Design review of the part built by this model. Coordinates are the model's own, in mm. A direction names the side the tool comes from. Round coordinates to 2 decimals unless told otherwise and drop trailing zeros. Loops run counter-clockwise (first coordinate to the right, second up) from the corner with the lowest first, then second, coordinate; pieces in that order, holes last. Notation, with made-up numbers: (34.25, 84) - (74.25, 84) arc R17 cw to (74.25, 113) - close; hole circle Ø4 at (17.5, -40). An arc over 180 degrees is marked (long way). Return JSON: item names as keys, results as strings. Group by question number.
from build123d import *

# Parameters (mm, degrees)
MAIN_BODY_SKETCH_W            = 29
MAIN_BODY_SKETCH_H            = 11
MAIN_BODY_EXTRUDE_DEPTH       = 1.5
TILTED_OFFSHOOT_SKETCH_W      = 11
TILTED_OFFSHOOT_SKETCH_H      = 24
TILTED_OFFSHOOT_EXTRUDE_DEPTH = 1.5
F_2_7_2_7_DIAMETER_HOLE1_D    = 2.7
F_3_0_3_DIAMETER_HOLE1_D      = 3


with BuildPart() as part:
    # Main Body Sketch → Main Body Extrude (new body)
    with BuildSketch(Plane(origin=(0, 0, 0), x_dir=(1, 0, 0), z_dir=(0, 1, 0))):
        Polygon((-29, -11), (-29, 0), (-29, 2.5), (-47.33030278, 2.5), (-47.33030278, -13.5), (-29, -13.5), align=None)
        with Locations((-14.5, -5.5)):
            Rectangle(MAIN_BODY_SKETCH_W, MAIN_BODY_SKETCH_H)
        with BuildLine():
            ThreePointArc((-47.33030278, -13.5), (-49, -5.5), (-47.33030278, 2.5))
            Line((-47.33030278, 2.5), (-47.33030278, -13.5))
        make_face()
    extrude(amount=MAIN_BODY_EXTRUDE_DEPTH)

    # Tilted Offshoot Sketch → Tilted Offshoot Extrude (add)
    with BuildSketch(Plane(origin=(0, 0, 0), x_dir=(0, 0, 1), z_dir=(-0.707106781, 0.707106781, 0))):
        with Locations((5.5, 12)):
            Rectangle(TILTED_OFFSHOOT_SKETCH_W, TILTED_OFFSHOOT_SKETCH_H)
    extrude(amount=TILTED_OFFSHOOT_EXTRUDE_DEPTH)

    # Ø2.7 (2.7) Diameter Hole1 (through all)
    with Locations(Plane(origin=(0, 1.5, 0), x_dir=(1, 0, 0), z_dir=(0, 1, 0))):
        with Locations((-45, -10.5), (-33, -0.5)):
            Hole(F_2_7_2_7_DIAMETER_HOLE1_D / 2)

    # Ø3.0 (3) Diameter Hole1 (through all)
    with Locations(Plane(origin=(-1.060660172, 1.060660172, 0), x_dir=(0.707106781, 0.707106781, 0), z_dir=(-0.707106781, 0.707106781, 0))):
        with Locations((20, -5.5)):
            Hole(F_3_0_3_DIAMETER_HOLE1_D / 2)


solid = part.part
Q1. Draft analysis for pull direction X (two halves, no side actions). For faces 1 (the flat face through (-29, 1, 12)), 2 (the flat face through (-4, 1, 0)), 3 (the cylindrical face through (-44.005, 0.74, 9.588)), state which applies: pulls with the +X half, pulls with the -X half, needs draft (parallel to the pull), parting line crosses it, or undercut.
Q2. Add section B-B, the plane y = 4.5. State the section outline as (x, z) points.
Q3. For line 1 (Z direction, x = -45, y = 0.4); line 2 (Z direction, x = -33, y = 0.45); line 3 (Y direction, x = -35, z = 8.5), list the stretches that pass through material, from the lowest coordinate up.
Q4. Tool access review of faces 4 (the flat face through (-29, 1, -1)), 5 (the flat face through (-25, 1.5, 5)), 6 (the flat face through (-38, 1, 13.5)), 7 (the flat face through (-3, 1, 11)): name each direction out of +Z, -Z, +X, -X, +Y, -Y from which nothing blocks a thin tool from reaching the whole face with its end or side.
Q5. Insertion check: pin 1 Ø6 at (y, z) = (12, 9.5) entering from +X; pin 2 Ø1.5 at (y, z) = (3.5, 7.5) entering from +X; pin 3 Ø1.2 at (y, z) = (1, -2) entering from +X. Each pin has a flat end and moves straight along its axis. Give the tip position at first contact, or say it passes through.
Q6. Add section C-C, the plane x = -8.5. State the section outline as (y, z) points.
Q7. Add section A-A, the plane x = -45. State the section outline as (y, z) points.
Evaluation:
{
 "1": {"face 1": "pulls with the +X half", "face 2": "needs draft", "face 3": "undercut"},
 "2": {"outline": "(2.38, 0) - (4.5, 0) - (4.5, 11) - (2.38, 11) - close"},
 "3": {"line 1": "-2.5 to 9.15, 11.85 to 13.5", "line 2": "-2.5 to -0.85, 1.85 to 13.5", "line 3": "0 to 1.5"},
 "4": {"face 4": "-Z, +X, +Y, -Y", "face 5": "+Z, -Z, -X, +Y", "face 6": "+Z, +X, -X, +Y, -Y", "face 7": "+Z, +X, +Y, -Y"},
 "5": {"pin 1": "x = 15", "pin 2": "x = 4.25", "pin 3": "x = -29"},
 "6": {"outline": "(0, 0) - (1.5, 0) - (1.5, 11) - (0, 11) - close"},
 "7": {"outline": "(0, -2.5) - (1.5, -2.5) - (1.5, 9.15) - (0, 9.15) - close; (0, 11.85) - (1.5, 11.85) - (1.5, 13.5) - (0, 13.5) - close"}
}
